from build123d import *

# Parameters (mm, degrees)
SKETCH1_R           = 24
SKETCH1_R_2         = 14
BOSS_EXTRUDE3_DEPTH = 14
BOSS_EXTRUDE7_START = 20
SKETCH5_R           = 14
BOSS_EXTRUDE7_DEPTH = 64
SKETCH7_R           = 12.5
BOSS_EXTRUDE8_DEPTH = 40


with BuildPart() as part:
    # Sketch1 → Boss-Extrude3 (new body, symmetric)
    with BuildSketch(Plane.XY):
        Circle(SKETCH1_R)
        Circle(SKETCH1_R_2, mode=Mode.SUBTRACT)
    extrude(amount=BOSS_EXTRUDE3_DEPTH, both=True)

    # Sketch5 → Boss-Extrude7 (add)
    with BuildSketch(Plane(origin=(0, 0, 0), x_dir=(0, 0, -1), z_dir=(1, 0, 0)).offset(BOSS_EXTRUDE7_START)):
        Circle(SKETCH5_R)
    extrude(amount=BOSS_EXTRUDE7_DEPTH)

    # Sketch7 → Boss-Extrude8 (add)
    with BuildSketch(Plane(origin=(84, 0, 0), x_dir=(0, 0, -1), z_dir=(1, 0, 0))):
        Circle(SKETCH7_R)
    extrude(amount=BOSS_EXTRUDE8_DEPTH)


solid = part.part
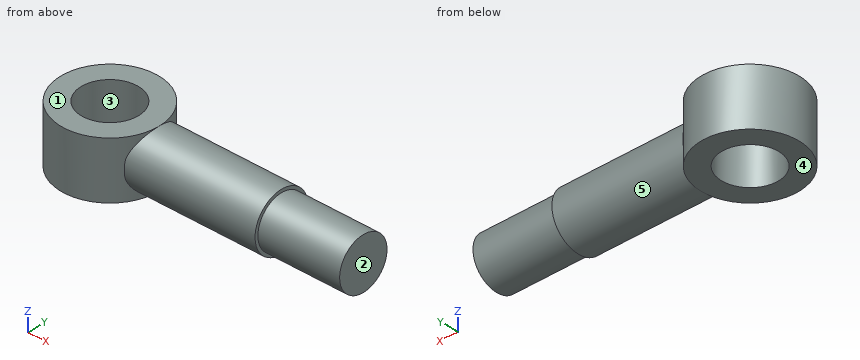
Part model, mm, in its own coordinate system. Face numbers are marked on the shaded views. A direction names the side the tool comes from. Give positions to 0.01 mm unless a question says otherwise; leave off trailing zeros. Order: outer loops, then holes, each group sorted by start corner. A loop starts at its lowest first (then second) coordinate and runs counter-clockwise, first axis right, second up. Notation, with made-up numbers: (24, 34) - (76, 34) arc R29 cw to (76, 72) - close; hole circle Ø8 at (78, 36.5). An arc over 180 degrees is marked (long way). Use a Markdown table: item, result.
1) Saw through at A-A on x = 0. List the corners of the cut face in (y, z).
Checked values:
| item | result |
|---|---|
| outline | (-24, -14) - (-14, -14) - (-14, 14) - (-24, 14) - close; (14, -14) - (24, -14) - (24, 14) - (14, 14) - close |
2) Two-plate mould, pull along X, no slides. Class the marked faces 1, 2 and 3: +X half, -X half, draft (parallel to the pull), parting line (faces both ways), or undercut.
Checked values:
| item | result |
|---|---|
| face 1 | draft |
| face 2 | +X half |
| face 3 | undercut |
3) Saw through at B-B on z = 0. List the corners of the cut face in (x, y).
Checked values:
| item | result |
|---|---|
| outline | (20, -14) - (84, -14) - (84, -12.5) - (124, -12.5) - (124, 12.5) - (84, 12.5) - (84, 14) - (20, 14) - (20, 13.27) arc R24 ccw (long way) to (20, -13.27) - close; hole circle Ø28 at (0, 0) |
4) Saw through at C-C on y = -8. List the corners of the cut face in (x, z).
Checked values:
| item | result |
|---|---|
| outline | (-22.63, -14) - (-11.49, -14) - (-11.49, 14) - (-22.63, 14) - close; (11.49, -14) - (22.63, -14) - (22.63, -11.49) - (84, -11.49) - (84, -9.6) - (124, -9.6) - (124, 9.6) - (84, 9.6) - (84, 11.49) - (22.63, 11.49) - (22.63, 14) - (11.49, 14) - close |
5) Flat gauge pins, fed straight in: P1, Ø1, axis at x = 2, z = -4.5, coming from the +Y side; P2, Ø1, axis at y = -3.5, z = -2.5, coming from the -X side; P3, Ø2, axis at x = 89.5, z = -11, coming from the +Y side. Where does each tip first touch, or does it go through?
Checked values:
| item | result |
|---|---|
| P1 | y = 23.95 |
| P2 | x = -23.81 |
| P3 | y = 7.5 |
6) Probe L1, parallel to Y at x = 0, z = -6.25; L2, parallel to X at y = 9.5, z = 9.5; L3, parallel to X at y = 9, z = 11. List the from-to ranges inside material, lowest first. Write a range as from..to.
Checked values:
| item | result |
|---|---|
| L1 | -24..-14, 14..24 |
| L2 | -22.04..-10.28, 10.28..84 |
| L3 | -22.25..-10.72, 10.72..22.25 |
7) Saw through at D-D on x = 63.5. List the corners of the cut face in (y, z), plus the area to 3 significant figures.
Checked values:
| item | result |
|---|---|
| outline | circle Ø28 at (0, 0) |
| area | 616 mm² |
8) 3-axis set-ups, long thin cutter, end or side, ignore diameter. For the marked faces 4 and 5: which of +Z, -Z, +X, -X, +Y, -Y reach the whole face in a straight line?
Checked values:
| item | result |
|---|---|
| face 4 | -Z, +X, -X, +Y, -Y |
| face 5 | +X |
